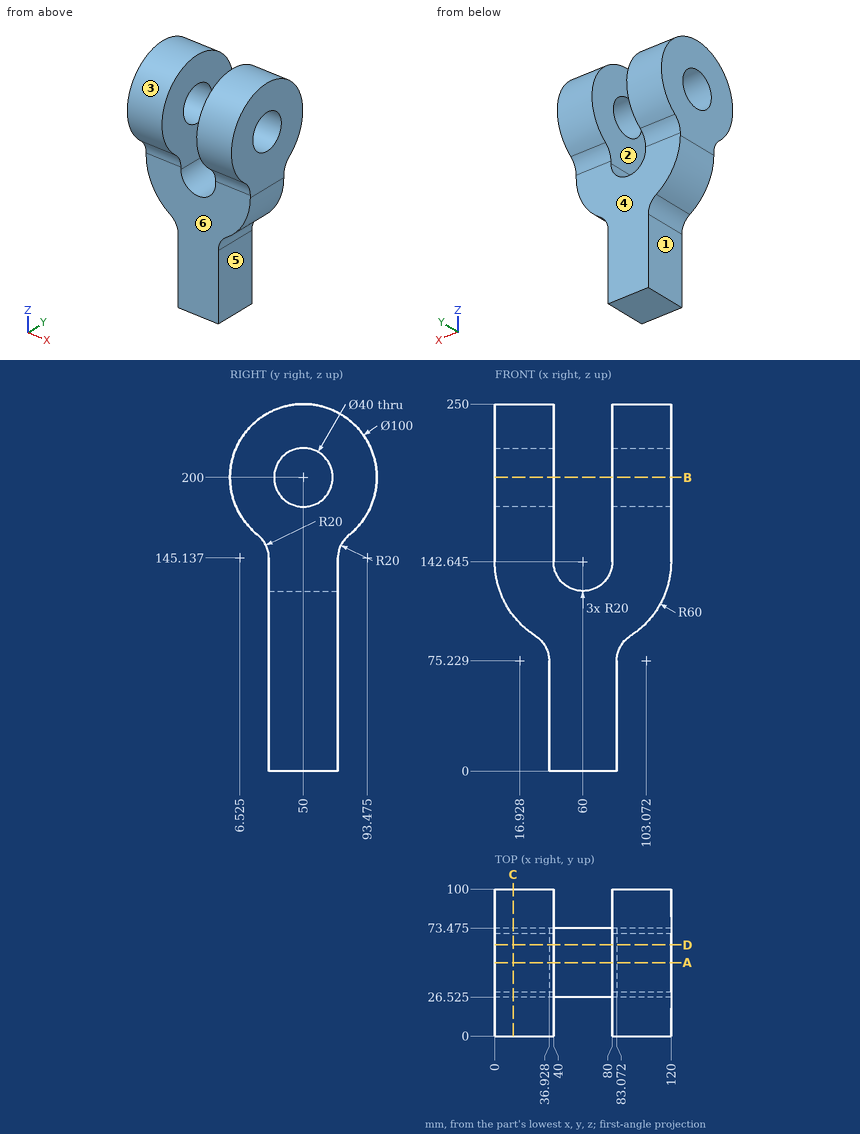
Answer from the drawing. Dimensions are ordinates in mm from the lowest x, y and z of the part. A direction names the side the tool comes from. Round coordinates to 2 decimals unless told otherwise and drop trailing zeros. Loops run counter-clockwise (first coordinate to the right, second up) from the corner with the lowest first, then second, coordinate; pieces in that order, holes last.
1) For the marked faces 4, 5 and 6, determine the directions among +Z, -Z, +X, -X, +Y, -Y from which every point of the face is accessible in a straight line to the end or side of a thin tool.
Outcome:
face 4: -Z, +X, -X, +Y
face 5: -Z, +X, +Y, -Y
face 6: -Z, +X, -X, -Y
2) A cutting plane is placed at D-D on y = 62. Determine the outline of the cut face in (x, z) (1 decimal), plus the area to 3 significant figures.
Outcome:
outline: (0, 142.6) arc R60 ccw to (27.7, 92.1) arc R20 cw to (36.9, 75.2) - (36.9, 0) - (83.1, 0) - (83.1, 75.2) arc R20 cw to (92.3, 92.1) arc R60 ccw to (120, 142.6) - (120, 184) - (80, 184) - (80, 142.6) arc R20 cw to (40, 142.6) - (40, 184) - (0, 184) - close; (0, 216) - (40, 216) - (40, 248.5) - (0, 248.5) - close; (80, 216) - (120, 216) - (120, 248.5) - (80, 248.5) - close
area: 14,900 mm2
3) Consider line 1 (X direction, y = 26, z = 222.5); line 2 (Y direction, x = 25, z = 200); line 3 (Y direction, x = 67.5, z = 17) (1 decimal). Determine where each line is inside the solid, lowest interval first.
Outcome:
line 1: x = 0 to 40, 80 to 120
line 2: y = 0 to 30, 70 to 100
line 3: y = 26.5 to 73.5
4) Given P1, Ø12, axis at x = 26, y = 51, coming from the +Z side; P2, Ø5, axis at x = 82, y = 59, coming from the +Z side; P3, Ø6, axis at x = 107.5, z = 222, coming from the -Y side; P4, Ø6, axis at x = 56, y = 30.5, coming from the -Z side, each flat-ended and moving along its own axis, determine where each tip first touches the part or whether it passes through.
Outcome:
P1: stops at z = 250
P2: stops at z = 249.58
P3: stops at y = 3.75
P4: stops at z = 0
5) A cutting plane is placed at C-C on x = 12.5. Determine the outline of the cut face in (y, z) (1 decimal), plus the area to 4 significant figures.
Outcome:
outline: (18.9, 160.8) arc R20 cw to (26.5, 145.1) - (26.5, 106) - (73.5, 106) - (73.5, 145.1) arc R20 cw to (81.1, 160.8) arc R50 ccw (long way) to start; hole circle Ø40 at (50, 200)
area: 8,785 mm2
6) A cutting plane is placed at A-A on y = 50. Determine the outline of the cut face in (x, z) (1 decimal), plus the area to 3 significant figures.
Outcome:
outline: (0, 142.6) arc R60 ccw to (27.7, 92.1) arc R20 cw to (36.9, 75.2) - (36.9, 0) - (83.1, 0) - (83.1, 75.2) arc R20 cw to (92.3, 92.1) arc R60 ccw to (120, 142.6) - (120, 180) - (80, 180) - (80, 142.6) arc R20 cw to (40, 142.6) - (40, 180) - (0, 180) - close; (0, 220) - (40, 220) - (40, 250) - (0, 250) - close; (80, 220) - (120, 220) - (120, 250) - (80, 250) - close
area: 14,300 mm2
7) A cutting plane is placed at B-B on z = 200. Determine the outline of the cut face in (x, y), plus the area to 3 significant figures.
Outcome:
outline: (0, 0) - (40, 0) - (40, 30) - (0, 30) - close; (0, 70) - (40, 70) - (40, 100) - (0, 100) - close; (80, 0) - (120, 0) - (120, 30) - (80, 30) - close; (80, 70) - (120, 70) - (120, 100) - (80, 100) - close
area: 4,800 mm2
8) For a pull along X with two mould halves and no side action, classify the marked faces 1, 2 and 3 as released by +X, released by -X, zero draft, split by the parting line, or undercut.
Outcome:
face 1: released by -X
face 2: undercut
face 3: zero draft
